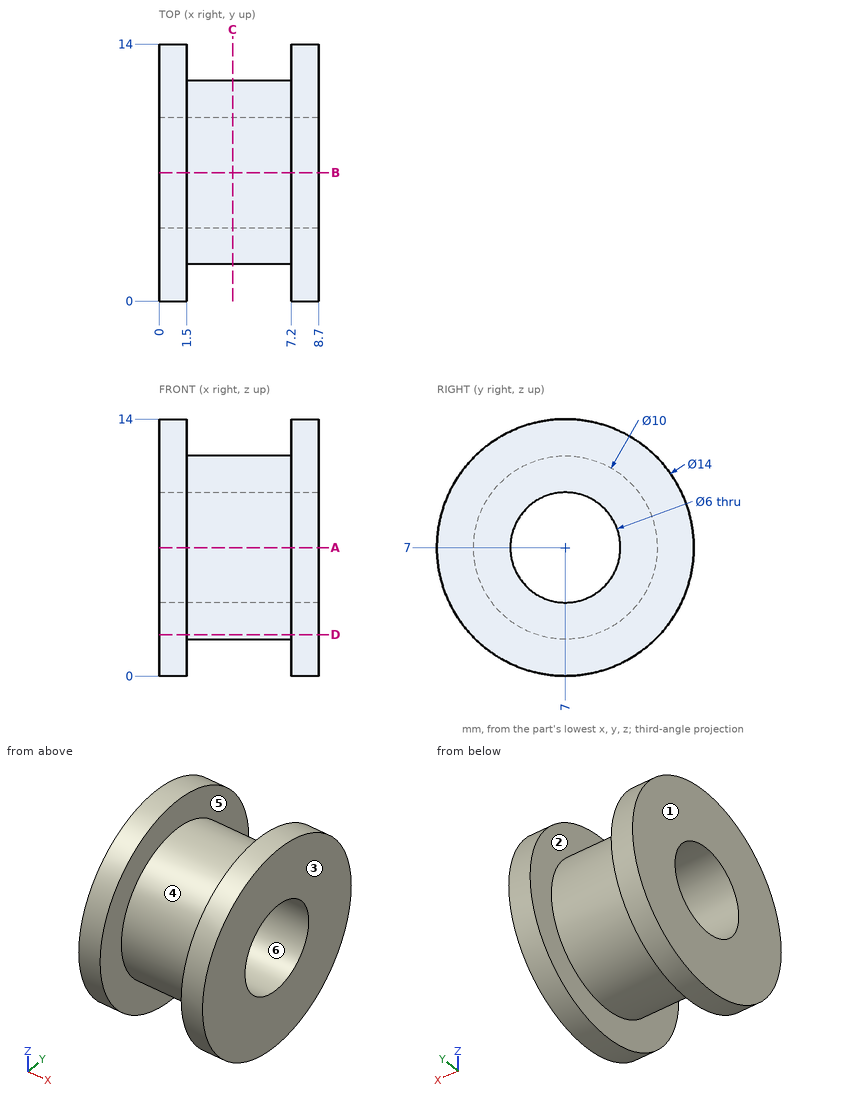
Could you check a few things on this drawing? It's one solid part, dimensions in mm from its lowest x, y, z. A direction names the side the tool comes from. Round coordinates to 2 decimals unless told otherwise and drop trailing zeros. Order: outer loops, then holes, each group sorted by start corner. A loop starts at its lowest first (then second) coordinate and runs counter-clockwise, first axis right, second up. Notation, with made-up numbers: M -6,54.5 L -2,54.5 A15 cw -2,59.5 Z; hole C -24,-38 d10. An arc over 180 degrees is marked long. Return JSON: item names as keys, results as strings. Group by question number.
1. I'm going to push flat-ended pins straight in: pin 1 Ø5 at (x, z) = (6.5, 12.5) entering from -Y; pin 2 Ø1.5 at (x, y) = (5.5, 9) entering from -Z; pin 3 Ø4 at (x, y) = (1, 9.5) entering from -Z. Where does each tip first touch, or does it pass through?
2. On a 3-axis mill with a long thin cutter (end or side, diameter ignored), from which of +Z, -Z, +X, -X, +Y, -Y can I reach the whole of each face in a straight line? I mean the marked faces 5 and 6. Say none if no direction works.
3. If we mould it in two halves opening along X, with no side actions, what happens to the marked faces 1, 2, 3 and 4? For each: pulls with the +X half, pulls with the -X half, needs draft (parallel to the pull), parting line crosses it, or undercut.
4. If we section it at A-A on z = 7: List the corners of the cut face in (x, y) for me.
5. If we section it at C-C on x = 4: List the corners of the cut face in (y, z) for me.
6. Please list where these lines run through material, in increasing order: probe 1 along Y at (x, z) = (5.5, 7); probe 2 along X at (y, z) = (7.5, 1); probe 3 along Y at (x, z) = (7.5, 4.25).
7. If we section it at D-D on z = 2.25: List the corners of the cut face in (x, y) for me.
Reply:
{
 "1": {"pin 1": "y = 0.72", "pin 2": "z = 2.16", "pin 3": "z = 0.02"},
 "2": {"face 5": "none", "face 6": "+X, -X"},
 "3": {"face 1": "pulls with the -X half", "face 2": "undercut", "face 3": "pulls with the +X half", "face 4": "undercut"},
 "4": {"outline": "M 0,0 L 1.5,0 L 1.5,2 L 7.2,2 L 7.2,0 L 8.7,0 L 8.7,4 L 0,4 Z; M 0,10 L 8.7,10 L 8.7,14 L 7.2,14 L 7.2,12 L 1.5,12 L 1.5,14 L 0,14 Z"},
 "5": {"outline": "C 7,7 d10; hole C 7,7 d6"},
 "6": {"probe 1": "2 to 4, 10 to 12", "probe 2": "0 to 1.5, 7.2 to 8.7", "probe 3": "0.56 to 5.8, 8.2 to 13.44"},
 "7": {"outline": "M 0,1.86 L 1.5,1.86 L 1.5,5.44 L 7.2,5.44 L 7.2,1.86 L 8.7,1.86 L 8.7,12.14 L 7.2,12.14 L 7.2,8.56 L 1.5,8.56 L 1.5,12.14 L 0,12.14 Z"}
}
